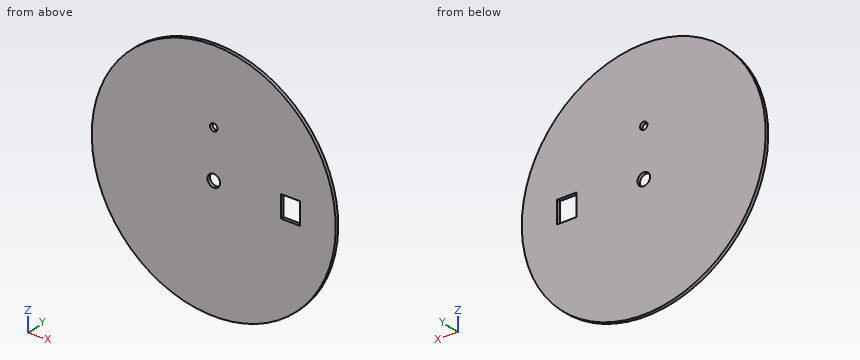
from build123d import *

# Parameters (mm, degrees)
SKETCH1_R           = 16.5
BOSS_EXTRUDE1_DEPTH = 0.44
SKETCH2_R           = 0.85
CUT_EXTRUDE1_DEPTH  = 0.44
SKETCH3_R           = 0.5
SKETCH3_W           = 2.6
SKETCH3_H           = 3
CUT_EXTRUDE4_DEPTH  = 0.44


with BuildPart() as part:
    # Sketch1 → Boss-Extrude1 (new body)
    with BuildSketch(Plane(origin=(0, 0, 0), x_dir=(1, 0, 0), z_dir=(0, 1, 0))):
        with Locations(Location((0, 0, 0), (0, 0, 270))):
            Circle(SKETCH1_R)
    extrude(amount=BOSS_EXTRUDE1_DEPTH)

    # Sketch2 → Cut-Extrude1 (cut)
    with BuildSketch(Plane(origin=(0, 0.44, 0), x_dir=(1, 0, 0), z_dir=(0, 1, 0))):
        with Locations(Location((0, 0, 0), (0, 0, 270))):
            Circle(SKETCH2_R)
    extrude(amount=-CUT_EXTRUDE1_DEPTH, mode=Mode.SUBTRACT)

    # Sketch3 → Cut-Extrude4 (cut)
    with BuildSketch(Plane(origin=(0, 0.44, 0), x_dir=(1, 0, 0), z_dir=(0, 1, 0))):
        with Locations(Location((0, -6.5, 0), (0, 0, 270))):
            Circle(SKETCH3_R)
        with Locations((10.4, 0)):
            Rectangle(SKETCH3_W, SKETCH3_H)
    extrude(amount=-CUT_EXTRUDE4_DEPTH, mode=Mode.SUBTRACT)


solid = part.part
Could you check a few things on this model? Use its own coordinates, in mm. Give positions to 0.01 mm unless a question says otherwise; leave off trailing zeros. Order: outer loops, then holes, each group sorted by start corner. A loop starts at its lowest first (then second) coordinate and runs counter-clockwise, first axis right, second up.
Item 1: If we section it at B-B, the plane z = 0: Write out the boundary of the cut face in (x, y), plus the area to 3 significant figures.
Item 2: If we section it at D-D, the plane z = 6.5: Write out the boundary of the cut face in (x, y).
Item 3: I need wall thicknesses on line 1 (X direction, y = 0.25, z = 0); line 2 (Z direction, x = 9.5, y = 0.2); line 3 (Z direction, x = -5.5, y = 0.4). Which ranges of each line are inside material? Lowest first, please.
Item 4: If we section it at A-A, the plane x = 0: Write out the boundary of the cut face in (y, z), plus the area to 3 significant figures.
Item 5: If we section it at C-C, the plane y = 0.3: Write out the boundary of the cut face in (x, z), plus the area to 3 significant figures.
Item 6: I'm going to push flat-ended pins straight in: pin 1 (1.4 mm diameter, centred on x = 0, z = 0, fed in from -Y); pin 2 (8 mm diameter, centred on x = -1, z = -2, fed in from -Y). Where does each tip first touch, or does it pass through?
Values:
1. outline: (-16.5, 0) - (-0.85, 0) - (-0.85, 0.44) - (-16.5, 0.44) - close; (0.85, 0) - (9.1, 0) - (9.1, 0.44) - (0.85, 0.44) - close; (11.7, 0) - (16.5, 0) - (16.5, 0.44) - (11.7, 0.44) - close
1. area: 12.6 mm2
2. outline: (-15.17, 0) - (-0.5, 0) - (-0.5, 0.44) - (-15.17, 0.44) - close; (0.5, 0) - (15.17, 0) - (15.17, 0.44) - (0.5, 0.44) - close
3. line 1: x = -16.5 to -0.85, 0.85 to 9.1, 11.7 to 16.5
3. line 2: z = -13.49 to -1.5, 1.5 to 13.49
3. line 3: z = -15.56 to 15.56
4. outline: (0, -16.5) - (0.44, -16.5) - (0.44, -0.85) - (0, -0.85) - close; (0, 0.85) - (0.44, 0.85) - (0.44, 6) - (0, 6) - close; (0, 7) - (0.44, 7) - (0.44, 16.5) - (0, 16.5) - close
4. area: 13.3 mm2
5. outline: circle Ø33 at (0, 0); hole circle Ø1.7 at (0, 0); hole circle Ø1 at (0, 6.5); hole (9.1, -1.5) - (11.7, -1.5) - (11.7, 1.5) - (9.1, 1.5) - close
5. area: 844 mm2
6. pin 1: passes through
6. pin 2: stops at y = 0
